Answer from the drawing. Dimensions are ordinates in mm from the lowest x, y and z of the part. Round coordinates to 2 decimals unless told otherwise and drop trailing zeros. Order: outer loops, then holes, each group sorted by start corner. A loop starts at its lowest first (then second) coordinate and runs counter-clockwise, first axis right, second up. Notation, with made-up numbers: (40.5, 62.25) - (73.5, 62.25) arc R20 cw to (73.5, 88.25) - close; hole circle Ø11 at (-13, 62.5). An arc over 180 degrees is marked (long way). One line per question, with ' | ' between items. Start each with the question number.
1) A flat-ended cylindrical pin translates along its axis: pin 1 (5 mm diameter, centred on x = 38.5, y = 118.5, fed in from -Z). Find the tip coordinate at first contact, or state that the pin passes through.
2) Straight lines are drawn through the part: line 1 (Y direction, x = 100, z = 7.75); line 2 (Y direction, x = 25, z = 3.25). For each, find the intervals that lie inside material, in ascending order. Write a range as from..to.
3) The part is cut by section A-A, the plane x = 25. Give the vertices of the cut face in (y, z), plus the area to 3 significant figures.
4) The part is cut by section C-C, the plane z = 1.5. Give the vertices of the cut face in (x, y).
5) The part is cut by section B-B, the plane y = 100. Give the vertices of the cut face in (x, z), plus the area to 3 significant figures.
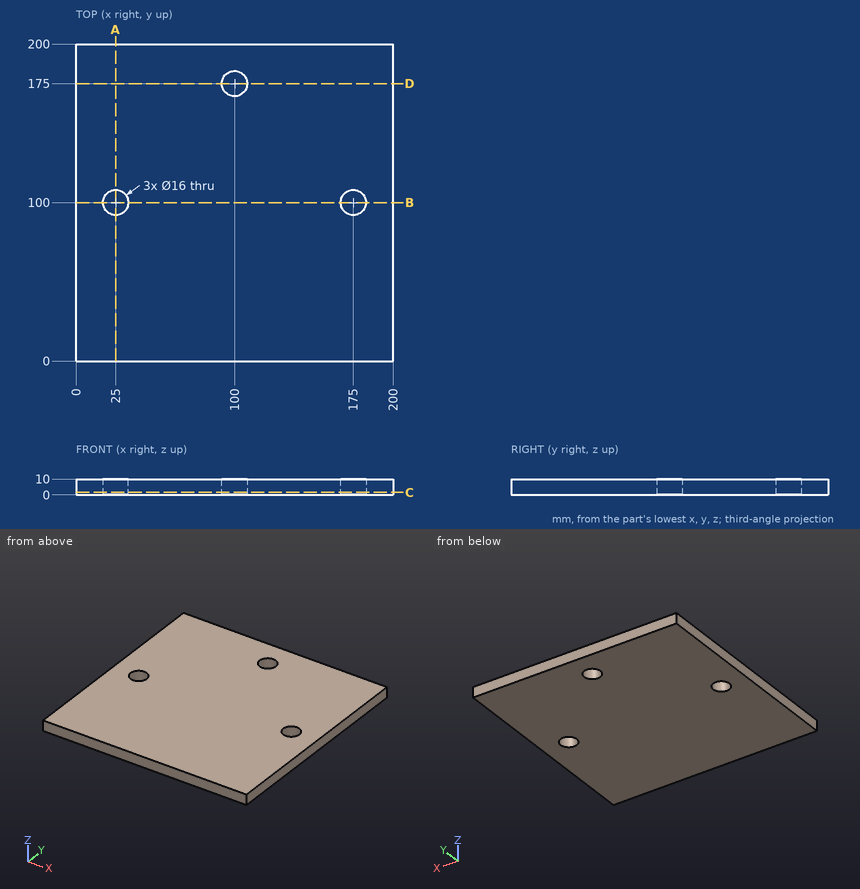
Values:
1) pin 1: stops at z = 0
2) line 1: y = 0..167, 183..200 | line 2: y = 0..92, 108..200
3) outline: (0, 0) - (92, 0) - (92, 10) - (0, 10) - close; (108, 0) - (200, 0) - (200, 10) - (108, 10) - close | area: 1,840 mm^2
4) outline: (0, 0) - (200, 0) - (200, 200) - (0, 200) - close; hole circle Ø16 at (25, 100); hole circle Ø16 at (100, 175); hole circle Ø16 at (175, 100)
5) outline: (0, 0) - (17, 0) - (17, 10) - (0, 10) - close; (33, 0) - (167, 0) - (167, 10) - (33, 10) - close; (183, 0) - (200, 0) - (200, 10) - (183, 10) - close | area: 1,680 mm^2
